Here's how the part is built. I have some questions about the finished solid (model axes, mm). A direction names the side the tool comes from. Round coordinates to 2 decimals unless told otherwise and drop trailing zeros. Loops run counter-clockwise (first coordinate to the right, second up) from the corner with the lowest first, then second, coordinate; pieces in that order, holes last. Notation, with made-up numbers: M 55.25,-36 L 76.25,-36 A12 ccw 76.25,-15 Z; hole C 30,52.5 d4. An arc over 180 degrees is marked long. Answer as a JSON object with one key per item and string values.
from build123d import *

# Parameters (mm, degrees)
F1_DEPTH = 6
F2_DEPTH = 1


with BuildPart() as f1:
    # F0 (on Top) → F1 (new body)
    with BuildSketch(Plane.XY):
        Polygon((-25, 0), (-19.9713055044, 0), (-19.9713055044, 3.5559397656), (-24.9629596584, 3.5559397656), align=None)
        Polygon((-40, 0), (-25, 0), (-24.9629596584, 3.5559397656), (-40, 3.5559397656), align=None)
        with BuildLine():
            Line((-24.9629596584, 3.5559397656), (-19.9713055044, 3.5559397656))
            Line((-19.9713055044, 3.5559397656), (-19.9713055044, 6))
            Line((-19.9713055044, 6), (-23.9375011772, 6))
            ThreePointArc((-23.9375011772, 6), (-24.2340866143, 5.2892201799), (-24.9479170826, 5.000054247))
            Line((-24.9479170826, 5.000054247), (-24.9629596584, 3.5559397656))
        make_face()
        with BuildLine():
            Line((-19.9713055044, 8.8996905833), (-19.9713055044, 12))
            Line((-19.9713055044, 12), (-24.9375011772, 12))
            Line((-24.9375011772, 12), (-24.9375011772, 7))
            ThreePointArc((-24.9375011772, 7), (-24.230394396, 6.7071067812), (-23.9375011772, 6))
            Line((-23.9375011772, 6), (-19.9713055044, 6))
            Line((-19.9713055044, 6), (-19.9713055044, 8.8996905833))
        make_face()
        with BuildLine():
            Line((-40, 3.5559397656), (-24.9629596584, 3.5559397656))
            Line((-24.9629596584, 3.5559397656), (-24.9479170826, 5.000054247))
            ThreePointArc((-24.9479170826, 5.000054247), (-25.6482809973, 5.2965854371), (-25.9375011772, 6))
            Line((-25.9375011772, 6), (-40, 6))
            Line((-40, 6), (-40, 3.5559397656))
        make_face()
        with BuildLine():
            Line((-24.9375011772, 7), (-24.9375011772, 12))
            Line((-24.9375011772, 12), (-40, 12))
            Line((-40, 12), (-40, 6))
            Line((-40, 6), (-25.9375011772, 6))
            ThreePointArc((-25.9375011772, 6), (-25.6446079584, 6.7071067812), (-24.9375011772, 7))
        make_face()
    extrude(amount=F1_DEPTH)

    # F0 (on Top) → F2 (join)
    with BuildSketch(Plane.XY):
        Polygon((-19.9713055044, 0), (0, 0), (0, 12), (-19.9713055044, 12), (-19.9713055044, 8.8996905833), (-2.2525554523, 8.8996905833), (-2.2525554523, 3.5559397656), (-19.9713055044, 3.5559397656), align=None)
    extrude(amount=F2_DEPTH)


solid = f1.part
Item 1: For faces 1 (the face through (-25, 0, 2)), 2 (the face through (-10, 3, 1)), 3 (the face through (-2.253, 6.3, 0.5)), which set-ups out of +Z, -Z, +X, -X, +Y, -Y let a thin tool reach every point of the face, with its end or its side?
Solution:
{"face 1": "+Z, -Z, +X, -X, -Y", "face 2": "+Z, +X, +Y, -Y", "face 3": "+Z, -Z"}
Item 2: I want a section at A-A on z = 3.25. List the corners of the cut face in (x, y) for me.
Solution:
{"outline": "M -40,0 L -19.97,0 L -19.97,12 L -40,12 Z; hole C -24.94,6 d2"}
Item 3: I want a section at D-D on z = 0.4. List the corners of the cut face in (x, y) for me.
Solution:
{"outline": "M -40,0 L 0,0 L 0,12 L -40,12 Z; hole C -24.94,6 d2; hole M -19.97,3.56 L -2.25,3.56 L -2.25,8.9 L -19.97,8.9 Z"}
Item 4: I want a section at C-C on y = 4.5. List the corners of the cut face in (x, z) for me, plus the area to 3 significant figures.
Solution:
{"outline": "M -40,0 L -19.97,0 L -19.97,6 L -40,6 Z; M -2.25,0 L 0,0 L 0,1 L -2.25,1 Z", "area": "122 mm2"}
Item 5: For P1, Ø1.8, axis at y = 5.5, z = 2.5, coming from the +X side; P2, Ø4, axis at x = -33.5, y = 8.5, coming from the -Z side; P3, Ø6, axis at x = -7.5, y = 2.5, coming from the +Z side, each with a flat end and sliding along its axis, tell me the tip position at first contact or that it passes through.
Solution:
{"P1": "stops at x = -19.97", "P2": "stops at z = 0", "P3": "stops at z = 1"}
Item 6: If I drill on L1, parallel to Y at x = -25, z = 0.6; L2, parallel to Y at x = -4, z = 0.7; L3, parallel to Z at x = -3.5, y = 1.5, over which ranges is the centre line in solid material (lowest first)? Write a range as from..to.
Solution:
{"L1": "y = 0..5, 7..12", "L2": "y = 0..3.56, 8.9..12", "L3": "z = 0..1"}
Item 7: I want a section at B-B on x = -19. List the corners of the cut face in (y, z) for me.
Solution:
{"outline": "M 0,0 L 3.56,0 L 3.56,1 L 0,1 Z; M 8.9,0 L 12,0 L 12,1 L 8.9,1 Z"}
Item 8: We'd pull the mould along Y, two halves only. Please class faces 4 (the face through (-11.2, 8.9, 0.5)), 5 (the face through (-29, 12, 2)), 6 (the face through (-24.7, 4.8, 0)), 7 (the face through (-11, 3.556, 0.5)): +Y half, -Y half, draft (parallel to the pull), parting line (faces both ways), or undercut.
Solution:
{"face 4": "undercut", "face 5": "+Y half", "face 6": "draft", "face 7": "undercut"}
